Autodesk Inventor part; units mm, degrees
ref_plane "YZ Plane" through (0, 0, 0) normal (1, 0, 0) x (0, 1, 0)
ref_plane "XZ Plane" through (0, 0, 0) normal (0, 1, 0) x (-1, 0, 0)
ref_plane "XY Plane" through (0, 0, 0) normal (0, 0, 1) x (1, 0, 0)
sketch "Sketch1" plane through (0, 0, 0) normal (0, 0, 1) x (1, 0, 0)
  circle A0 centre (0, 0) radius 33 construction
  circle A1 centre (0, 0) radius 19.1
  line L0 (-101, -32.5) -> (29, -32.5)
  line L1 (29, -32.5) -> (29, 32.5)
  line L2 (29, 32.5) -> (-101, 32.5)
  line L3 (-101, 32.5) -> (-101, -32.5)
  line L4 (-101, -32.5) -> (29, 32.5) construction
  line L5 (29, -32.5) -> (-101, 32.5) construction
  line L6 (-101, 0) -> (29, 0) construction
  arc A2 (-91, 23) -> (-91, 17) centre (-91, 20) ccw
  line L7 (-91, 20) -> (-49, 20) construction
  arc A3 (-52, 20) -> (-49, 17) centre (-49, 20) ccw construction
  line L8 (-91, 23) -> (-49, 23)
  line L9 (-91, 17) -> (-49, 17)
  arc A4 (-88, 20) -> (-91, 23) centre (-91, 20) ccw construction
  arc A5 (-91, 17) -> (-88, 20) centre (-91, 20) ccw construction
  arc A6 (-49, 23) -> (-52, 20) centre (-49, 20) ccw construction
  arc A7 (-49, 17) -> (-49, 23) centre (-49, 20) ccw
  arc A8 (-91, -17) -> (-91, -23) centre (-91, -20) ccw
  line L10 (-91, -23) -> (-49, -23)
  line L11 (-91, -17) -> (-49, -17)
  arc A9 (-49, -23) -> (-49, -17) centre (-49, -20) ccw
  line L12 (23.3345, -23.3345) -> (-23.3345, 23.3345) construction
  line L13 (-23.3345, -23.3345) -> (23.3345, 23.3345) construction
  circle A10 centre (23.3345, 23.3345) radius 3
  circle A11 centre (-23.3345, 23.3345) radius 3
  circle A12 centre (-23.3345, -23.3345) radius 3
  circle A13 centre (23.3345, -23.3345) radius 3
  point P0 (-36, 0)
  dimension "d0" = 66
  dimension "d1" = 38.2
  dimension "d2" = 130
  dimension "d3" = 65
  dimension "d4" = 101
  dimension "d5" = 6
  dimension "d6" = 10
  dimension "d7" = 52
  dimension "d8" = 40
  dimension "d9" = 45
extrude "Plate1" add sketch "Sketch1" along normal blind 4.75
fillet "Corner Round1" radius 6 4 edges at (29, 32.5, 2.375) (29, -32.5, 2.375) (-101, -32.5, 2.375) (-101, 32.5, 2.375)
equation "\"BendRadius\" = Thickness"
equation "\"BendReliefWidth\" = Thickness"
equation "\"BendReliefDepth\" = 0.5 * Thickness"
equation "\"CornerReliefSize\" = 4 * Thickness"
equation "\"MinimumRemnant\" = 2 * Thickness"
equation "\"TransitionRadius\" = BendRadius"
equation "\"JacobiRadiusSize\" = BendRadius"
equation "\"GapSize\" = Thickness"
equation "\"d10\" = BendRadius"
properties part number "nema_support_1" material "Steel, Carbon"
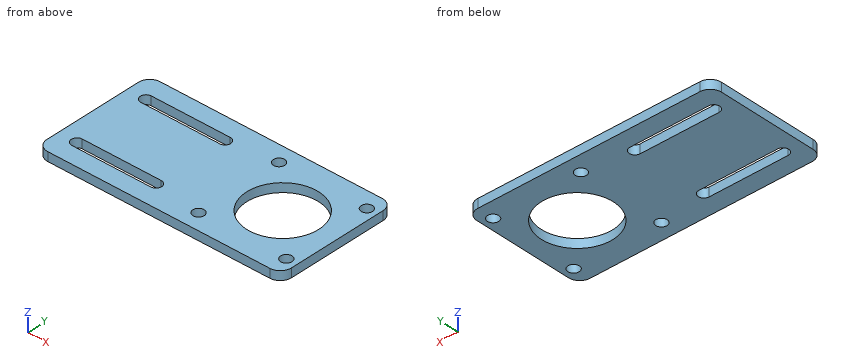
Input: part model. Units: mm. Frame: model coordinates. Coordinates: 2 decimals unless noted, no trailing zeros. Loops run counter-clockwise (first coordinate to the right, second up) from the corner with the lowest first, then second, coordinate; pieces in that order, holes last. Notation, with made-up numbers: M -8,43.25 L -2,43.25 A10 ccw -2,51.25 Z; hole C 27,79 d1. An arc over 180 degrees is marked long. Use a Markdown table: item, result. Add a question column.
1) Section B-B, the plane x = 0. Return the cut outline in (y, z), plus the area to 3 significant figures.
2) Section C-C, the plane x = -47.5. Return the cut outline in (y, z).
3) Pin query (flat end, axial travel): P1, Ø7, axis at x = -23.33, y = -23.33, coming from the +Z side. Return the tip coordinate at first contact, or that it passes through.
4) Line query: L1, parallel to Y at x = -82, z = 0.4; L2, parallel to X at y = -26, z = 1.3; L3, parallel to Y at x = -24, z = 1.6. Output: solid intervals per line, ascending. Write a range as from..to.
5) Section A-A, the plane y = 0. Return the cut outline in (x, z).
6) Section D-D, the plane z = 2.15. Return the cut outline in (x, y), plus the area to 3 significant figures.
Answer below:
| question | item | result |
|---|---|---|
| 1 | outline | M -32.5,0 L -19.1,0 L -19.1,4.75 L -32.5,4.75 Z; M 19.1,0 L 32.5,0 L 32.5,4.75 L 19.1,4.75 Z |
| 1 | area | 127 mm2 |
| 2 | outline | M -32.5,0 L -22.6,0 L -22.6,4.75 L -32.5,4.75 Z; M -17.4,0 L 17.4,0 L 17.4,4.75 L -17.4,4.75 Z; M 22.6,0 L 32.5,0 L 32.5,4.75 L 22.6,4.75 Z |
| 3 | P1 | z = 4.75 |
| 4 | L1 | -32.5..-23, -17..17, 23..32.5 |
| 4 | L2 | -101..-24.71, -21.96..21.96, 24.71..29 |
| 4 | L3 | -32.5..-26.26, -20.41..20.41, 26.26..32.5 |
| 5 | outline | M -101,0 L -19.1,0 L -19.1,4.75 L -101,4.75 Z; M 19.1,0 L 29,0 L 29,4.75 L 19.1,4.75 Z |
| 6 | outline | M -101,-26.5 A6 ccw -95,-32.5 L 23,-32.5 A6 ccw 29,-26.5 L 29,26.5 A6 ccw 23,32.5 L -95,32.5 A6 ccw -101,26.5 Z; hole M -91,-23 L -49,-23 A3 ccw -49,-17 L -91,-17 A3 ccw Z; hole M -91,17 L -49,17 A3 ccw -49,23 L -91,23 A3 ccw Z; hole C -23.33,-23.33 d6; hole C -23.33,23.33 d6; hole C 0,0 d38.2; hole C 23.33,-23.33 d6; hole C 23.33,23.33 d6 |
| 6 | area | 6,600 mm2 |
